The listing builds one solid part. Answer for the finished solid, in the listing's coordinates (mm). A direction names the side the tool comes from. Give positions to 0.01 mm unless a question says otherwise; leave off trailing zeros. Order: outer loops, then holes, each group sorted by start corner. A loop starts at its lowest first (then second) coordinate and runs counter-clockwise, first axis right, second up. Notation, with made-up numbers: (26, -38.75) - (73, -38.75) arc R22 cw to (73, -32.75) - close; hole circle Ø4 at (66.5, -20.5). An arc over 180 degrees is marked (long way). Use a Markdown table: item, result. Add a question column.
1) Straight lines are drawn through the part: line 1 (X direction, y = -10, z = -19.25); line 2 (X direction, y = -5, z = 16.5); line 3 (Y direction, x = -22.5, z = -21). For each, find the intervals that lie inside material, in ascending order.
2) The mould has two halves that part along X. Classify faces 1 (the face through (-30, -10, -20)), 2 (the face through (30, -10, -21)), 3 (the face through (-25.55, -8.74, -20.43)): released by +X, released by -X, zero draft, split by the parting line, or undercut.
3) Find section B-B, the plane x = 22.5. Determine the outline of the cut face in (y, z).
4) Find section C-C, the plane y = -11. Determine the outline of the cut face in (x, z).
5) Find section A-A, the plane z = 22.5. Determine the outline of the cut face in (x, y).
6) Find section D-D, the plane y = -17. Determine the outline of the cut face in (x, z).
7) For faces 4 (the face through (1.058, -10, 21)), 5 (the face through (-8, -10, 25.5)), 6 (the face through (26, -10, -15.5)), 7 (the face through (-15, -10, 5)), determine the directions among +Z, -Z, +X, -X, +Y, -Y from which every point of the face is accessible in a straight line to the end or side of a thin tool.
8) Flat-ended cylindrical pins translate along their axes: pin 1 (4 mm diameter, centred on y = -10, z = 5.5, fed in from -X); pin 2 (10 mm diameter, centred on y = -8.5, z = 6, fed in from +X); pin 3 (1 mm diameter, centred on x = -17.5, y = -10.5, fed in from +Z); pin 4 (8 mm diameter, centred on x = 17.5, y = -4, fed in from +Z). Find the tip coordinate at first contact, or state that the pin passes through.
from build123d import *

# Parameters (mm, degrees)
F1_DEPTH = 20
F3_D     = 6.6
F4_D     = 6.6


with BuildPart() as f1:
    # F0 (on Front) → F1 (new body)
    with BuildSketch(Plane.XZ):
        with BuildLine():
            Line((-30, -25.5), (30, -25.5))
            Line((30, -25.5), (30, -15.5))
            Line((30, -15.5), (15, -15.5))
            Line((15, -15.5), (15, 25.5))
            Line((15, 25.5), (1.057532, 25.5))
            Line((1.057532, 25.5), (1.057532, 15.443924))
            ThreePointArc((1.057532, 15.443924), (-0.053951, -4.499854), (-0.950175, 15.454756))
            Line((-0.950175, 15.454756), (-0.950175, 25.5))
            Line((-0.950175, 25.5), (-15, 25.5))
            Line((-15, 25.5), (-15, -10.487244))
            Line((-15, -10.487244), (-15, -15.5))
            Line((-15, -15.5), (-30, -15.5))
            Line((-30, -15.5), (-30, -25.5))
        make_face()
    extrude(amount=F1_DEPTH)

    # F3 (through all)
    with Locations(Plane(origin=(0, 0, -25.5), x_dir=(1, 0, 0), z_dir=(0, 0, -1))):
        with Locations((-22.5, 10)):
            Hole(F3_D / 2)

    # F4 (through all)
    with Locations(Plane(origin=(0, 0, -25.5), x_dir=(1, 0, 0), z_dir=(0, 0, -1))):
        with Locations((22.5, 10)):
            Hole(F4_D / 2)


solid = f1.part
The answers:
| question | item | result |
|---|---|---|
| 1 | line 1 | -30 to -25.8, -19.2 to 19.2, 25.8 to 30 |
| 1 | line 2 | -15 to -0.95, 1.06 to 15 |
| 1 | line 3 | -20 to -13.3, -6.7 to 0 |
| 2 | face 1 | released by -X |
| 2 | face 2 | released by +X |
| 2 | face 3 | undercut |
| 3 | outline | (-20, -25.5) - (-13.3, -25.5) - (-13.3, -15.5) - (-20, -15.5) - close; (-6.7, -25.5) - (0, -25.5) - (0, -15.5) - (-6.7, -15.5) - close |
| 4 | outline | (-30, -25.5) - (-25.64, -25.5) - (-25.64, -15.5) - (-30, -15.5) - close; (-19.36, -25.5) - (19.36, -25.5) - (19.36, -15.5) - (15, -15.5) - (15, 25.5) - (1.06, 25.5) - (1.06, 15.44) arc R10 cw (long way) to (-0.95, 15.45) - (-0.95, 25.5) - (-15, 25.5) - (-15, -15.5) - (-19.36, -15.5) - close; (25.64, -25.5) - (30, -25.5) - (30, -15.5) - (25.64, -15.5) - close |
| 5 | outline | (-15, -20) - (-0.95, -20) - (-0.95, 0) - (-15, 0) - close; (1.06, -20) - (15, -20) - (15, 0) - (1.06, 0) - close |
| 6 | outline | (-30, -25.5) - (30, -25.5) - (30, -15.5) - (15, -15.5) - (15, 25.5) - (1.06, 25.5) - (1.06, 15.44) arc R10 cw (long way) to (-0.95, 15.45) - (-0.95, 25.5) - (-15, 25.5) - (-15, -15.5) - (-30, -15.5) - close |
| 7 | face 4 | +Z, +Y, -Y |
| 7 | face 5 | +Z, +X, -X, +Y, -Y |
| 7 | face 6 | +Z, +X, +Y, -Y |
| 7 | face 7 | +Z, -X, +Y, -Y |
| 8 | pin 1 | x = -15 |
| 8 | pin 2 | x = 15 |
| 8 | pin 3 | z = -15.5 |
| 8 | pin 4 | z = 25.5 |
